```python
from build123d import *

# Parameters (mm, degrees)
F0_W     = 127
F0_H     = 35.7124
F0_R     = 1.5875
F0_R_2   = 4.6228
F0_R_3   = 2.0193
F1_DEPTH = 12.7


with BuildPart() as f1:
    # F0 (on Top) → F1 (new body)
    with BuildSketch(Plane.XY):
        with Locations((63.5, 17.8562)):
            Rectangle(F0_W, F0_H)
        with Locations((15.875, 17.8562)):
            Circle(F0_R, mode=Mode.SUBTRACT)
        with Locations((45.72, 17.8562)):
            Circle(F0_R_2, mode=Mode.SUBTRACT)
        with Locations((81.28, 17.8562)):
            Circle(F0_R_2, mode=Mode.SUBTRACT)
        with Locations((111.125, 17.8562)):
            Circle(F0_R, mode=Mode.SUBTRACT)
        with Locations((45.72, 17.8562)):
            Circle(F0_R_2)
        with Locations((45.72, 17.8562)):
            Circle(F0_R_3, mode=Mode.SUBTRACT)
        with Locations((81.28, 17.8562)):
            Circle(F0_R_2)
        with Locations((81.28, 17.8562)):
            Circle(F0_R_3, mode=Mode.SUBTRACT)
    extrude(amount=F1_DEPTH)


solid = f1.part
```
Can you work these out from the model? Positions are in its coordinate system, mm. Coordinates: 2 decimals unless noted, no trailing zeros. Loops run counter-clockwise (first coordinate to the right, second up) from the corner with the lowest first, then second, coordinate; pieces in that order, holes last. Notation, with made-up numbers: (34, 19) -> (52, 19) arc R24 cw to (52, 48) -> close; hole circle Ø7 at (-8, -2). An arc over 180 degrees is marked (long way). Answer as a JSON object with one key per item and string values.
1) For P1, Ø2, axis at x = 110.5, z = 8.5, coming from the -Y side, with a flat end and sliding along its axis, tell me the tip position at first contact or that it passes through.
Results:
{"P1": "stops at y = 0"}
2) Thinking about a two-plate mould opening in Y: for faces 1 (the face through (63, 35.712, 6)), 2 (the face through (15.531, 16.306, 6.261)), 3 (the face through (63, 18, 12.7)), which applies, pulls with the +Y half, pulls with the -Y half, needs draft (parallel to the pull), parting line crosses it, or undercut?
Results:
{"face 1": "pulls with the +Y half", "face 2": "undercut", "face 3": "needs draft"}
3) Imagine slicing it at A-A (x = 45.72). Please give me the cut outline in (y, z).
Results:
{"outline": "(0, 0) -> (15.84, 0) -> (15.84, 12.7) -> (0, 12.7) -> close; (19.88, 0) -> (35.71, 0) -> (35.71, 12.7) -> (19.88, 12.7) -> close"}
4) If I drill on line 1 (X direction, y = 18, z = 7.25); line 2 (Y direction, x = 81.28, z = 3.25); line 3 (Y direction, x = 16, z = 4.25), over which ranges is the centre line in solid material (lowest first)?
Results:
{"line 1": "x = 0 to 14.29, 17.46 to 43.71, 47.73 to 79.27, 83.29 to 109.54, 112.71 to 127", "line 2": "y = 0 to 15.84, 19.88 to 35.71", "line 3": "y = 0 to 16.27, 19.44 to 35.71"}
